Source: three-view drawing plus pictorial views. Frame: mm from the lowest corner of the part. A direction names the side the tool comes from. Give positions to 0.01 mm unless a question says otherwise; leave off trailing zeros. Loops run counter-clockwise (first coordinate to the right, second up) from the corner with the lowest first, then second, coordinate; pieces in that order, holes last.
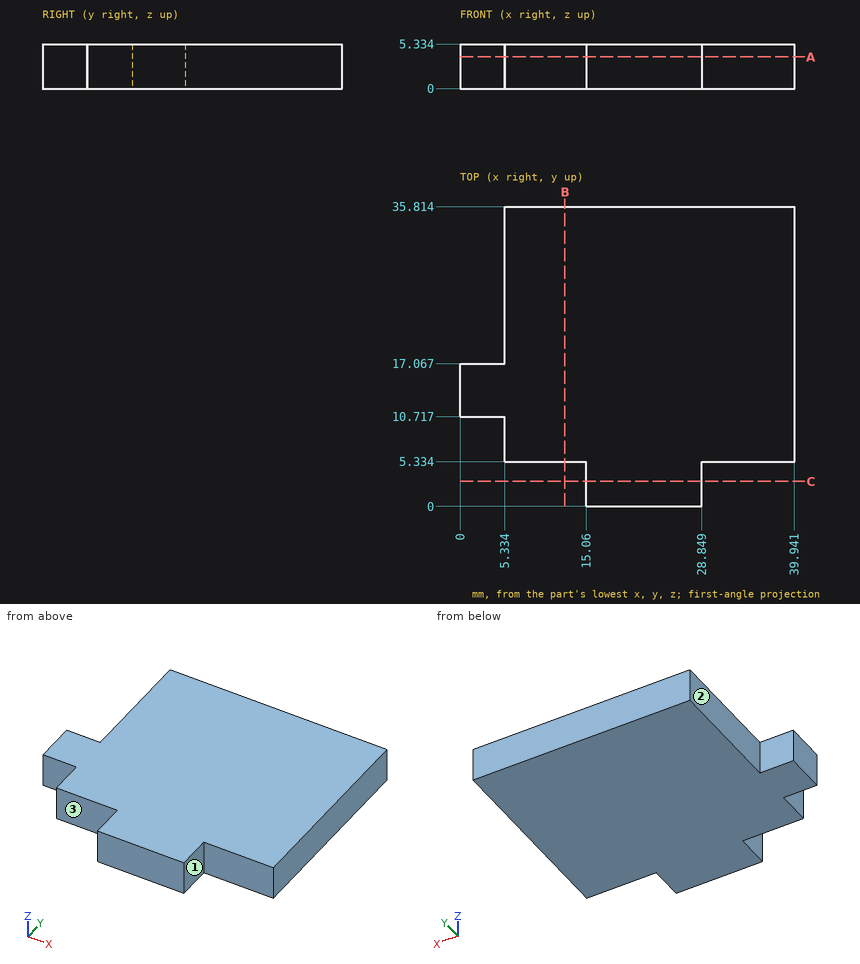
(1) Pin query (flat end, axial travel): pin 1 Ø2.5 at (y, z) = (23.5, 3.5) entering from -X; pin 2 Ø2.5 at (y, z) = (3.5, 2) entering from -X. Return the tip coordinate at first contact, or that it passes through.
Values follow:
pin 1: stops at x = 5.33
pin 2: stops at x = 15.06
(2) Cut plane B-B (x = 12.5). Return the cut outline in (y, z) (1 decimal).
Values follow:
outline: (5.3, 0) - (35.8, 0) - (35.8, 5.3) - (5.3, 5.3) - close
(3) Reachability of the marked faces 1, 2 and 3 from +Z, -Z, +X, -X, +Y, -Y: full face, straight path, thin tool, end or side. Return the list, or none.
Values follow:
face 1: +Z, -Z, +X, -Y
face 2: +Z, -Z, -X, +Y
face 3: +Z, -Z, -X, -Y
(4) Ray query, probe 1 along X at (y, z) = (2, 3.15); probe 2 along Y at (x, z) = (14, 1.65) (1 decimal); probe 3 along X at (y, z) = (34, 2.45) (1 decimal). Return the intervals inside material, ascending.
Values follow:
probe 1: x = 15.06 to 28.85
probe 2: y = 5.3 to 35.8
probe 3: x = 5.3 to 39.9
(5) Cut plane A-A (z = 3.8). Return the cut outline in (x, y) (1 decimal), and give its area (3 significant figures).
Values follow:
outline: (0, 10.7) - (5.3, 10.7) - (5.3, 5.3) - (15.1, 5.3) - (15.1, 0) - (28.8, 0) - (28.8, 5.3) - (39.9, 5.3) - (39.9, 35.8) - (5.3, 35.8) - (5.3, 17.1) - (0, 17.1) - close
area: 1,160 mm2
(6) Cut plane C-C (y = 3). Return the cut outline in (x, z) (1 decimal).
Values follow:
outline: (15.1, 0) - (28.8, 0) - (28.8, 5.3) - (15.1, 5.3) - close
